Input: part model. Units: mm. Frame: model coordinates. A direction names the side the tool comes from. Coordinates: 2 decimals unless noted, no trailing zeros. Loops run counter-clockwise (first coordinate to the right, second up) from the corner with the lowest first, then second, coordinate; pieces in that order, holes last.
Item 1: Section B-B on x = 0. Return loops of the section in (y, z).
Item 2: Ray query, line 1 along Y through (x, z) = (0, 0.5); line 2 along X through (y, z) = (0, 3.4); line 3 along X through (y, z) = (26, 3.8). Return the intervals inside material, ascending.
Item 3: Contact query for flat-ended pins moving along their axis: P1, Ø3, axis at x = -2, y = 1.5, coming from the +Z side; P2, Ø0.6, axis at x = 11.5, z = 6.5, coming from the +Y side. Output: stop coordinate, or through.
Item 4: Section D-D on y = -4.5. Return loops of the section in (x, z).
Item 5: Section C-C on z = 0.5. Give the number of separate pieces and of enclosed holes in the cut face, and give its area (3 significant figures).
Item 6: Reachability of faces 4 (the flat face through (-10, 13, 3)), 5 (the cylindrical face through (-1.08, 30.88, 3.96)) from +Z, -Z, +X, -X, +Y, -Y: full face, straight path, thin tool, end or side. Return the list, or none.
Item 7: Pull-direction query (X, two-part tool) for faces 1 (the cylindrical face through (14, 30, 4)), 2 (the cylindrical face through (-1.08, 4.88, 3.96)), 3 (the cylindrical face through (-8, -11, 3)); classes: released by +X, released by -X, zero draft, split by the parting line, or undercut.
Item 8: Section A-A on y = 13. Return loops of the section in (x, z).
Autodesk Inventor part; units mm, degrees
ref_plane "YZ Plane" through (0, 0, 0) normal (1, 0, 0) x (0, 1, 0)
ref_plane "XZ Plane" through (0, 0, 0) normal (0, 1, 0) x (-1, 0, 0)
ref_plane "XY Plane" through (0, 0, 0) normal (0, 0, 1) x (1, 0, 0)
sketch "S-SupportBase" plane through (0, 0, 0) normal (0, 0, 1) x (1, 0, 0)
  line L0 (0, 48) -> (0, -22) construction
  line L1 (0, 0) -> (20.5, 0) construction
  circle A0 centre (0, 0) radius 5
  circle A1 centre (0, 0) radius 3.15
  line L2 (0, -12) -> (20.5, -12)
  line L3 (20.5, -12) -> (20.5, 28)
  line L4 (20.5, 28) -> (13, 28)
  line L5 (13, 28) -> (13, 38)
  line L6 (13, 38) -> (-10, 38)
  line L7 (-10, 38) -> (-10, -12)
  line L8 (-10, -12) -> (0, -12)
  circle A2 centre (0, 26) radius 5
  circle A3 centre (0, 26) radius 3.15
  circle A4 centre (9.0936, 13) radius 7.5
  line L9 (8.9816, -0.1589) -> (15.0717, -0.1589) construction
  line L10 (15.0717, -0.1589) -> (15.0717, -6.2589) construction
  line L11 (15.0717, -6.2589) -> (8.9816, -6.2589) construction
  line L12 (8.9816, -6.2589) -> (8.9816, -0.1589) construction
  line L13 (15.2496, -6.2589) -> (13.386, -6.2589)
  line L14 (13.386, -6.2589) -> (11.6905, -4.0196)
  line L15 (11.6905, -4.0196) -> (11.1368, -4.0196)
  line L16 (11.1368, -4.0196) -> (11.1368, -6.2589)
  line L17 (11.1368, -6.2589) -> (9.6143, -6.2589)
  line L18 (9.6143, -6.2589) -> (9.6143, -0.1589)
  line L19 (9.6143, -0.1589) -> (12.0662, -0.1589)
  spline S0 degree 2 poles (12.0662, -0.1589) (12.5753, -0.1589) (13.3267, -0.2875) (13.648, -0.4852) knots 0 0 0 1 2 2 2
  spline S1 degree 2 poles (13.648, -0.4852) (13.9743, -0.6928) (14.3598, -1.3404) (14.3598, -1.8347) knots 0 0 0 1 2 2 2
  spline S2 degree 2 poles (14.3598, -1.8347) (14.3598, -2.5317) (13.7271, -3.4067) (13.1982, -3.6637) knots 0 0 0 1 2 2 2
  line L20 (13.1982, -3.6637) -> (15.2496, -6.2589)
  spline S3 degree 2 poles (12.7879, -2.0275) (12.7879, -1.7952) (12.6099, -1.464) (12.4072, -1.375) knots 0 0 0 1 2 2 2
  spline S4 degree 2 poles (12.4072, -1.375) (12.2639, -1.3157) (11.9129, -1.2811) (11.6509, -1.2811) knots 0 0 0 1 2 2 2
  line L21 (11.6509, -1.2811) -> (11.1368, -1.2811)
  line L22 (11.1368, -1.2811) -> (11.1368, -2.9222)
  line L23 (11.1368, -2.9222) -> (11.5768, -2.9222)
  spline S5 degree 2 poles (11.5768, -2.9222) (11.8931, -2.9222) (12.343, -2.8431) (12.4962, -2.7196) knots 0 0 0 1 2 2 2
  spline S6 degree 2 poles (12.4962, -2.7196) (12.6445, -2.6009) (12.7879, -2.2846) (12.7879, -2.0275) knots 0 0 0 1 2 2 2
  dimension "d0" = 20.5
  dimension "d1" = 10
  dimension "d2" = 6.3
  dimension "d3" = 12
  dimension "d4" = 10
  dimension "d5" = 40
  dimension "d6" = 10
  dimension "d9" = 26
  dimension "d14" = 23
  dimension "d20" = 15
extrude "Ex-Base1" add sketch "S-SupportBase" along normal blind 1 contours A0 | L8 L7 L6 L5 L4 L3 L2 | A2 | L13 L14 L15 L16 L17 L18 L19 S0 S1 S2 L20 | S6 S5 L23 L22 L21 S4 S3
extrude "Ex-Base2" add sketch "S-SupportBase" along normal blind 7 contours L8 L7 L6 L5 L4 L3 L2 | L13 L14 L15 L16 L17 L18 L19 S0 S1 S2 L20 | S6 S5 L23 L22 L21 S4 S3
fillet "Rundung1" radius 5 6 edges at (-10, -12, 3.5) (-10, 38, 3.5) (13, 38, 3.5) (13, 28, 3.5) (20.5, 28, 3.5) (20.5, -12, 3.5)
extrude "Extrusion3" cut sketch "S-SupportBase" against normal blind 0.5 from surface at 7 contours L13 L14 L15 L16 L17 L18 L19 S0 S1 S2 L20
properties part number "xy Motor Support Right for 4040 extra"
Results found:
1. outline: (-12, 0) - (-3.15, 0) - (-3.15, 1) - (-5, 1) - (-5, 7) - (-12, 7) - close; (3.15, 0) - (22.85, 0) - (22.85, 1) - (21, 1) - (21, 7) - (5, 7) - (5, 1) - (3.15, 1) - close; (29.15, 0) - (38, 0) - (38, 7) - (31, 7) - (31, 1) - (29.15, 1) - close
2. line 1: y = -12 to -3.15, 3.15 to 22.85, 29.15 to 38
2. line 2: x = -10 to -5, 5 to 20.5
2. line 3: x = -10 to -5, 5 to 19.72
3. P1: stops at z = 1
3. P2: stops at y = 36.84
4. outline: (-10, 0) - (20.5, 0) - (20.5, 7) - (13.86, 7) - (13.86, 6.5) - (12.05, 6.5) - (12.05, 7) - (11.14, 7) - (11.14, 6.5) - (9.61, 6.5) - (9.61, 7) - (2.18, 7) - (2.18, 1) - (-2.18, 1) - (-2.18, 7) - (-10, 7) - close
5. separate pieces: 1
5. enclosed holes: 3
5. area: 1,190 mm2
6. face 4: +Z, -Z, -X, +Y, -Y
6. face 5: +Z
7. face 1: released by +X
7. face 2: undercut
7. face 3: released by -X
8. outline: (-10, 0) - (1.59, 0) - (1.59, 7) - (-10, 7) - close; (16.59, 0) - (20.5, 0) - (20.5, 7) - (16.59, 7) - close
